```python
from build123d import *

# Parameters (mm, degrees)
SKETCH1_R           = 45
BOSS_EXTRUDE1_DEPTH = 15
SKETCH2_R           = 38.75
CUT_EXTRUDE1_DEPTH  = 14.5
SKETCH3_R           = 35
CUT_EXTRUDE2_DEPTH  = 66.270590621
BOSS_EXTRUDE2_START = -5
SKETCH4_R           = 65
SKETCH4_R_2         = 45
BOSS_EXTRUDE2_DEPTH = 5
SKETCH5_R           = 5
CUT_EXTRUDE3_DEPTH  = 93.466210045


with BuildPart() as part:
    # Sketch1 → Boss-Extrude1 (new body)
    with BuildSketch(Plane.XY):
        Circle(SKETCH1_R)
    extrude(amount=BOSS_EXTRUDE1_DEPTH)

    # Sketch2 → Cut-Extrude1 (cut)
    with BuildSketch(Plane.XY.offset(15)):
        Circle(SKETCH2_R)
    extrude(amount=-CUT_EXTRUDE1_DEPTH, mode=Mode.SUBTRACT)

    # Sketch3 → Cut-Extrude2 (cut, through all)
    with BuildSketch(Plane.XY.offset(0.5)):
        Circle(SKETCH3_R)
    extrude(amount=-CUT_EXTRUDE2_DEPTH, mode=Mode.SUBTRACT)

    # Sketch4 → Boss-Extrude2 (add)
    with BuildSketch(Plane.XY.offset(15).offset(BOSS_EXTRUDE2_START)):
        Circle(SKETCH4_R)
        Circle(SKETCH4_R_2, mode=Mode.SUBTRACT)
    extrude(amount=BOSS_EXTRUDE2_DEPTH)

    # Sketch5 → Cut-Extrude3 (cut, through all)
    with BuildSketch(Plane(origin=(0, 0, 10), x_dir=(-1, 0, 0), z_dir=(0, 0, -1))):
        with Locations((0, 55)):
            Circle(SKETCH5_R)
        with Locations((47.631397208, 27.5)):
            Circle(SKETCH5_R)
        with Locations((47.631397208, -27.5)):
            Circle(SKETCH5_R)
        with Locations((0, -55)):
            Circle(SKETCH5_R)
        with Locations((-47.631397208, -27.5)):
            Circle(SKETCH5_R)
        with Locations((-47.631397208, 27.5)):
            Circle(SKETCH5_R)
    extrude(amount=-CUT_EXTRUDE3_DEPTH, mode=Mode.SUBTRACT)


solid = part.part
```
The listing builds one solid part. Answer for the finished solid, in the listing's coordinates (mm). A direction names the side the tool comes from. Coordinates: 2 decimals unless noted, no trailing zeros. Loops run counter-clockwise (first coordinate to the right, second up) from the corner with the lowest first, then second, coordinate; pieces in that order, holes last. Notation, with made-up numbers: (47.5, -18.75) - (62.5, -18.75) arc R21 ccw to (62.5, -7.75) - close; hole circle Ø11 at (21.5, -26). An arc over 180 degrees is marked (long way). Use a Markdown table: item, result. Add a question column.
1) Find the intervals of material crossed by line 1 (Y direction, x = 49, z = 12); line 2 (Y direction, x = 0, z = 5.5); line 3 (Y direction, x = 0, z = 0.2), in increasing order.
2) The part is cut by section B-B, the plane x = 0. Give the vertices of the cut face in (y, z), and give its area (3 significant figures).
3) The part is cut by section A-A, the plane y = 0. Give the vertices of the cut face in (x, z), and give its area (3 significant figures).
4) The mould has two halves that part along Y. Classify faces 3 (the flat face through (-29, -20, 0.5)), 4 (the flat face through (28, -28, 15)), 5 (the cylindrical face through (-8.4, -37.83, 7.85)), 6 (the cylindrical face through (20.765, -39.923, 4.93)): released by +Y, released by -Y, zero draft, split by the parting line, or undercut.
5) For faces 1 (the flat face through (14, 44, 10)), 2 (the cylindrical face through (0.651, -50.043, 12.465)), determine the directions among +Z, -Z, +X, -X, +Y, -Y from which every point of the face is accessible in a straight line to the end or side of a thin tool.
6) The part is cut by section C-C, the plane z = 11.75. Give the vertices of the cut face in (x, y), and give its area (3 significant figures).
7) The part is cut by section D-D, the plane x = 24. Give the vertices of the cut face in (y, z).
8) Given pin 1 (1 mm diameter, centred on x = 3, z = 13, fed in from -Y); pin 2 (5 mm diameter, centred on y = 32.5, z = 8, fed in from +X); pin 3 (8 mm diameter, centred on y = -20, z = 5, fed in from +X), each flat-ended and moving along its own axis, determine where each tip first touches the part or whether it passes through.
Here are the results:
| question | item | result |
|---|---|---|
| 1 | line 1 | y = -42.71 to -32.31, -22.69 to 22.69, 32.31 to 42.71 |
| 1 | line 2 | y = -45 to -38.75, 38.75 to 45 |
| 1 | line 3 | y = -45 to -35, 35 to 45 |
| 2 | outline | (-65, 10) - (-60, 10) - (-60, 15) - (-65, 15) - close; (-50, 10) - (-45, 10) - (-45, 0) - (-35, 0) - (-35, 0.5) - (-38.75, 0.5) - (-38.75, 15) - (-50, 15) - close; (35, 0) - (45, 0) - (45, 10) - (50, 10) - (50, 15) - (38.75, 15) - (38.75, 0.5) - (35, 0.5) - close; (60, 10) - (65, 10) - (65, 15) - (60, 15) - close |
| 2 | area | 291 mm^2 |
| 3 | outline | (-65, 10) - (-45, 10) - (-45, 0) - (-35, 0) - (-35, 0.5) - (-38.75, 0.5) - (-38.75, 15) - (-65, 15) - close; (35, 0) - (45, 0) - (45, 10) - (65, 10) - (65, 15) - (38.75, 15) - (38.75, 0.5) - (35, 0.5) - close |
| 3 | area | 391 mm^2 |
| 4 | face 3 | undercut |
| 4 | face 4 | zero draft |
| 4 | face 5 | undercut |
| 4 | face 6 | split by the parting line |
| 5 | face 1 | -Z |
| 5 | face 2 | +Z, -Z |
| 6 | outline | circle Ø130 at (0, 0); hole circle Ø10 at (-47.63, -27.5); hole circle Ø10 at (-47.63, 27.5); hole circle Ø77.5 at (0, 0); hole circle Ø10 at (0, -55); hole circle Ø10 at (0, 55); hole circle Ø10 at (47.63, -27.5); hole circle Ø10 at (47.63, 27.5) |
| 6 | area | 8,080 mm^2 |
| 7 | outline | (-60.41, 10) - (-38.07, 10) - (-38.07, 0) - (-25.48, 0) - (-25.48, 0.5) - (-30.42, 0.5) - (-30.42, 15) - (-60.41, 15) - close; (25.48, 0) - (38.07, 0) - (38.07, 10) - (60.41, 10) - (60.41, 15) - (30.42, 15) - (30.42, 0.5) - (25.48, 0.5) - close |
| 8 | pin 1 | stops at y = -64.95 |
| 8 | pin 2 | stops at x = 57.13 |
| 8 | pin 3 | stops at x = 42.06 |
